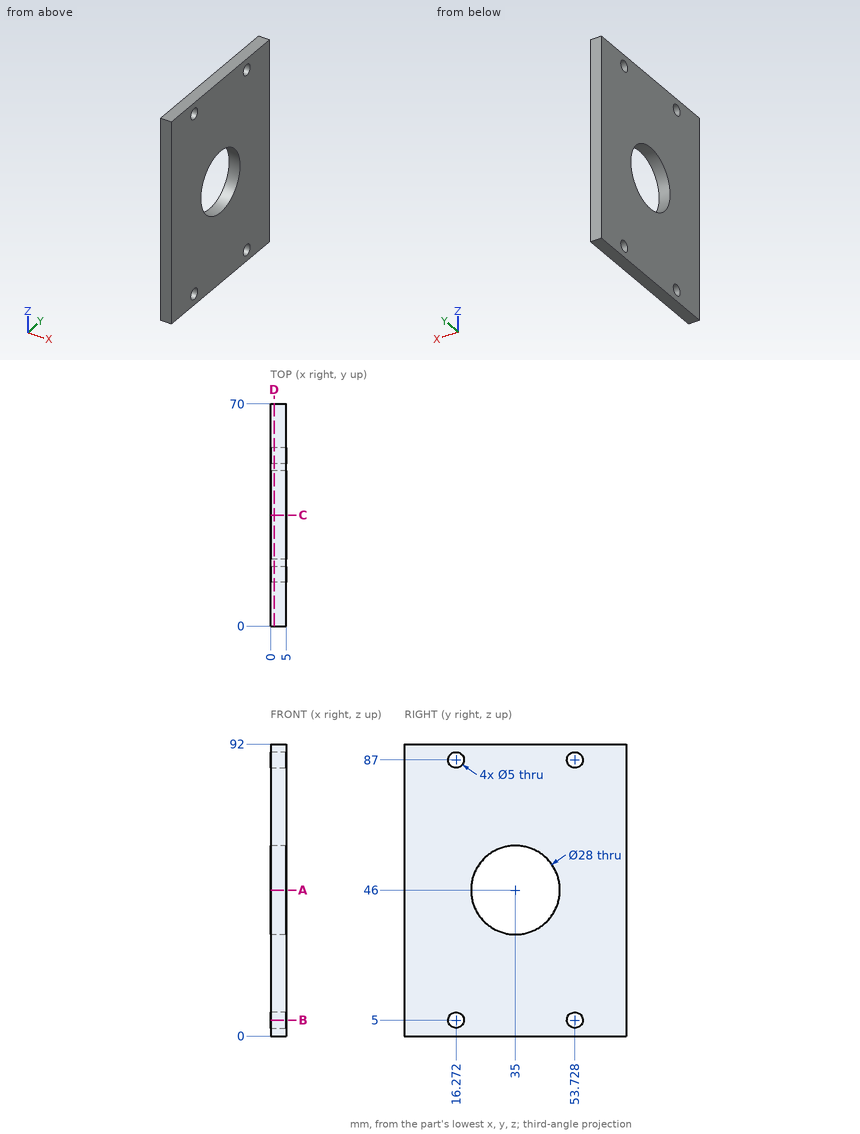
Print and shaded views of the part. All mm, measured from the part's lowest x, y and z. Coordinates: 2 decimals unless noted, no trailing zeros. Loops run counter-clockwise (first coordinate to the right, second up) from the corner with the lowest first, then second, coordinate; pieces in that order, holes last. Notation, with made-up numbers: (-33, 5) -> (-24, 5) arc R19 ccw to (-24, 37) -> close; hole circle Ø2 at (57, 3). An arc over 180 degrees is marked (long way). Use one line per item in the form item = value. Start each with the question number.
(1) Probe probe 1 along Y at (x, z) = (3.6, 87); probe 2 along Z at (x, y) = (4.2, 15); probe 3 along Y at (x, z) = (3.55, 46). List the from-to ranges inside material, lowest first. Write a range as from..to.
(2) Cut at A-A on z = 46. Give the cut face in (x, y).
(3) Cut at D-D on x = 1.15. Give the cut face in (y, z).
(4) Cut at C-C on y = 35. Give the cut face in (x, z), and give its area (3 significant figures).
(5) Cut at B-B on z = 5. Give the cut face in (x, y), and give its area (3 significant figures).
(6) Flat gauge pin, fed straight in: pin 1 (17 mm diameter, centred on y = 35, z = 46, fed in from -X). Where does the tip first touch, or does it go through?
Values:
q1.probe_1 = 0..13.77, 18.77..51.23, 56.23..70
q1.probe_2 = 0..2.85, 7.15..84.85, 89.15..92
q1.probe_3 = 0..21, 49..70
q2.outline = (0, 0) -> (5, 0) -> (5, 21) -> (0, 21) -> close; (0, 49) -> (5, 49) -> (5, 70) -> (0, 70) -> close
q3.outline = (0, 0) -> (70, 0) -> (70, 92) -> (0, 92) -> close; hole circle Ø5 at (16.27, 5); hole circle Ø5 at (16.27, 87); hole circle Ø28 at (35, 46); hole circle Ø5 at (53.73, 5); hole circle Ø5 at (53.73, 87)
q4.outline = (0, 0) -> (5, 0) -> (5, 32) -> (0, 32) -> close; (0, 60) -> (5, 60) -> (5, 92) -> (0, 92) -> close
q4.area = 320 mm2
q5.outline = (0, 0) -> (5, 0) -> (5, 13.77) -> (0, 13.77) -> close; (0, 18.77) -> (5, 18.77) -> (5, 51.23) -> (0, 51.23) -> close; (0, 56.23) -> (5, 56.23) -> (5, 70) -> (0, 70) -> close
q5.area = 300 mm2
q6.pin_1 = through
